Input: part model. Units: mm. Frame: model coordinates. Round coordinates to 2 decimals unless told otherwise and drop trailing zeros. Write each loop counter-clockwise with the first axis right and the second up, starting at its lowest first coordinate (ties: lowest second). Pieces come first, ordered by that corner, then holes. Notation, with made-up numbers: M 42,-6 L 77,-6 A8 ccw 77,9 Z; hole C 16,-35 d2. An arc over 180 degrees is marked long. Write each question's results on one line, items separated by ' | '. Start each with the question number.
```python
from build123d import *

# Parameters (mm, degrees)
SKETCH_W   = 600
SKETCH_H   = 120
SKETCH_R   = 14
SKETCH_W_2 = 34
SKETCH_H_2 = 34
PAD_DEPTH  = 15


with BuildPart() as part:
    # Sketch → Pad (new body)
    with BuildSketch(Plane.XY):
        with Locations((300, 60)):
            Rectangle(SKETCH_W, SKETCH_H)
        with Locations((80, 70)):
            Circle(SKETCH_R, mode=Mode.SUBTRACT)
        with Locations((450, 70)):
            Circle(SKETCH_R, mode=Mode.SUBTRACT)
        with Locations((150, 70)):
            Rectangle(SKETCH_W_2, SKETCH_H_2, mode=Mode.SUBTRACT)
        with Locations((520, 70)):
            Rectangle(SKETCH_W_2, SKETCH_H_2, mode=Mode.SUBTRACT)
    extrude(amount=PAD_DEPTH)


solid = part.part
```
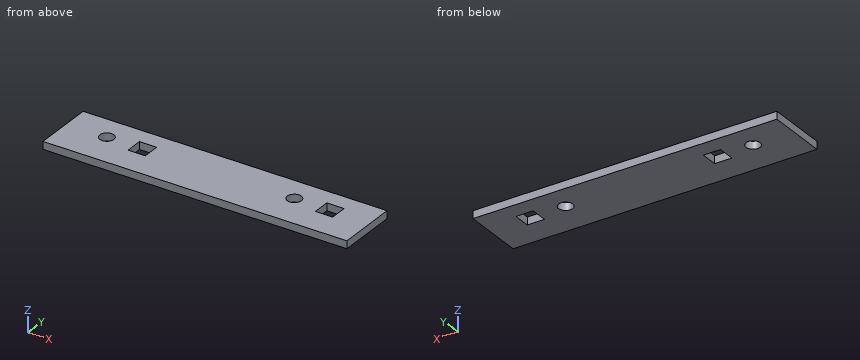
1. Line query: L1, parallel to X at y = 86.5, z = 4.75; L2, parallel to X at y = 68.5, z = 10.25; L3, parallel to Y at x = 450, z = 3.5. Output: solid intervals per line, ascending. Write a range as from..to.
2. Cut plane C-C on y = 70. Output: boundary loops of the cut face in (x, z).
3. Cut plane A-A on x = 80. Output: boundary loops of the cut face in (y, z), and give its area (3 significant figures).
4. Cut plane D-D on x = 156.5. Output: boundary loops of the cut face in (y, z), and give its area (3 significant figures).
5. Cut plane B-B on z = 9.5. Output: boundary loops of the cut face in (x, y).
Answers follow:
1) L1: x = 0..133, 167..503, 537..600 | L2: x = 0..66.08, 93.92..133, 167..436.08, 463.92..503, 537..600 | L3: y = 0..56, 84..120
2) outline: M 0,0 L 66,0 L 66,15 L 0,15 Z; M 94,0 L 133,0 L 133,15 L 94,15 Z; M 167,0 L 436,0 L 436,15 L 167,15 Z; M 464,0 L 503,0 L 503,15 L 464,15 Z; M 537,0 L 600,0 L 600,15 L 537,15 Z
3) outline: M 0,0 L 56,0 L 56,15 L 0,15 Z; M 84,0 L 120,0 L 120,15 L 84,15 Z | area: 1,380 mm2
4) outline: M 0,0 L 53,0 L 53,15 L 0,15 Z; M 87,0 L 120,0 L 120,15 L 87,15 Z | area: 1,290 mm2
5) outline: M 0,0 L 600,0 L 600,120 L 0,120 Z; hole C 80,70 d28; hole M 133,53 L 167,53 L 167,87 L 133,87 Z; hole C 450,70 d28; hole M 503,53 L 537,53 L 537,87 L 503,87 Z
